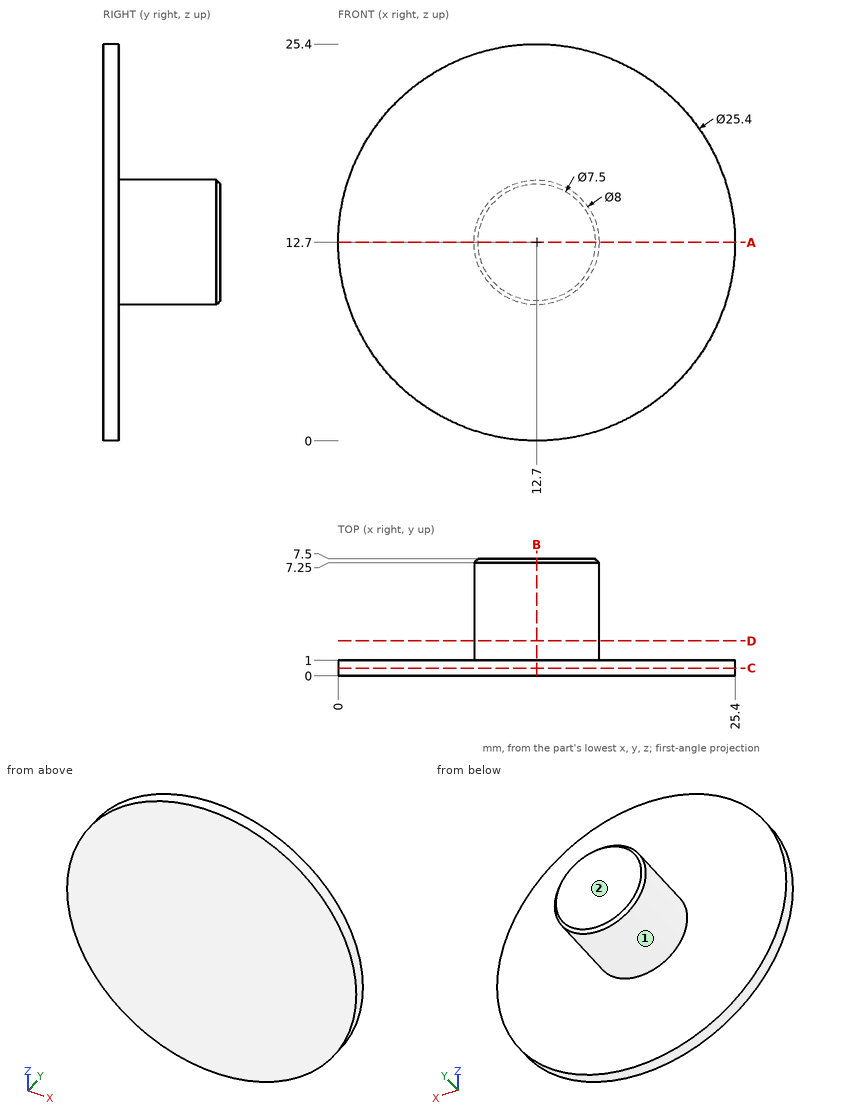
Here's the drawing with two shaded views (mm, measured from the low corner). I have some questions. A direction names the side the tool comes from. Round coordinates to 2 decimals unless told otherwise and drop trailing zeros. Order: outer loops, then holes, each group sorted by start corner. A loop starts at its lowest first (then second) coordinate and runs counter-clockwise, first axis right, second up. Notation, with made-up numbers: M 2,61 L 18,61 A27 cw 18,99 Z; hole C 49,42.5 d10. An arc over 180 degrees is marked long. Answer in a Markdown table with one row per item.
Item 1: Imagine slicing it at A-A, the plane z = 12.7. Write out the boundary of the cut face in (x, y), and give its area (3 significant figures).
A:
| item | result |
|---|---|
| outline | M 0,0 L 25.4,0 L 25.4,1 L 16.7,1 L 16.7,7.25 L 16.45,7.5 L 8.95,7.5 L 8.7,7.25 L 8.7,1 L 0,1 Z |
| area | 77.3 mm2 |
Item 2: Imagine slicing it at D-D, the plane y = 2.25. Write out the boundary of the cut face in (x, z), and give its area (3 significant figures).
A:
| item | result |
|---|---|
| outline | C 12.7,12.7 d8 |
| area | 50.3 mm2 |
Item 3: If I drill on L1, parallel to Y at x = 16.5, z = 19.25; L2, parallel to X at y = 0.75, z = 19.5; L3, parallel to X at y = 1.5, z = 10.5, over which ranges is the centre line in solid material (lowest first)? Write a range as from..to.
A:
| item | result |
|---|---|
| L1 | y = 0..1 |
| L2 | x = 1.97..23.43 |
| L3 | x = 9.36..16.04 |
Item 4: Imagine slicing it at C-C, the plane y = 0.5. Write out the boundary of the cut face in (x, z).
A:
| item | result |
|---|---|
| outline | C 12.7,12.7 d25.4 |
Item 5: For the marked faces 1 and 2, which set-ups out of +Z, -Z, +X, -X, +Y, -Y let a thin tool reach every point of the face, with its end or its side?
A:
| item | result |
|---|---|
| face 1 | +Y |
| face 2 | +Z, -Z, +X, -X, +Y |
Item 6: Imagine slicing it at B-B, the plane x = 12.7. Write out the boundary of the cut face in (y, z), and give its area (3 significant figures).
A:
| item | result |
|---|---|
| outline | M 0,0 L 1,0 L 1,8.7 L 7.25,8.7 L 7.5,8.95 L 7.5,16.45 L 7.25,16.7 L 1,16.7 L 1,25.4 L 0,25.4 Z |
| area | 77.3 mm2 |
